from build123d import *

# Parameters (mm, degrees)
BOSS_EXTRUDE1_DEPTH             = 24
SKETCH2_R                       = 4.125
BOSS_EXTRUDE2_DEPTH             = 10
CUT_EXTRUDE1_START              = -24
CUT_EXTRUDE1_DEPTH              = 1.5
CIRPATTERN1_COUNT               = 2
CIRPATTERN1_ANGLE               = 10
CIRPATTERN1_THE_OTHER_WAY_COUNT = 2
CIRPATTERN1_THE_OTHER_WAY_ANGLE = 10


with BuildPart() as part:
    # Sketch1 → Boss-Extrude1 (new body)
    with BuildSketch(Plane(origin=(0, 0, 0), x_dir=(1, 0, 0), z_dir=(0, 1, 0))):
        with BuildLine():
            ThreePointArc((-16.361099339, -0.997559555), (0, -2.429428688), (16.361258496, -0.999379302))
            ThreePointArc((16.361258496, -0.999379302), (19.819023, 3.925881002), (14.885248975, 7.371486655))
            ThreePointArc((14.885248975, 7.371486655), (0, 6.070571326), (-14.885089829, 7.373306345))
            ThreePointArc((-14.885089829, 7.373306345), (-19.808527535, 3.92587815), (-16.361099339, -0.997559555))
        make_face()
    extrude(amount=BOSS_EXTRUDE1_DEPTH)

    # Sketch2 → Boss-Extrude2 (add)
    with BuildSketch(Plane.XZ):
        with Locations(Location((-15.623094584, -3.187873395, 0), (0, 0, 90))):
            Circle(SKETCH2_R)
        with Locations(Location((15.633577289, -3.187873997, 0), (0, 0, 90))):
            Circle(SKETCH2_R)
    extrude(amount=BOSS_EXTRUDE2_DEPTH)

    # Sketch4 → Cut-Extrude1 (cut)
    with BuildSketch(Plane.XZ.offset(CUT_EXTRUDE1_START)):
        with BuildLine():
            Line((-2.1, 2.405913745), (-2.1, -6.140590357))
            ThreePointArc((-2.1, -6.140590357), (-0.000388897, -6.081612393), (2.1, -6.096161069))
            Line((2.1, -6.096161069), (2.1, 2.406147372))
            ThreePointArc((2.1, 2.406147372), (-3.4179e-05, 3.020482466), (-2.1, 2.405913745))
        make_face()
    cut_extrude1 = extrude(amount=CUT_EXTRUDE1_DEPTH, mode=Mode.SUBTRACT)

    # CirPattern1: Cut-Extrude1 ×2 about axis
    cirpattern1_axis = Axis((0.005241406, 24, -91.820571166), (0, 1, 0))
    for i in range(1, CIRPATTERN1_COUNT):
        add(cut_extrude1.rotate(cirpattern1_axis, i * CIRPATTERN1_ANGLE / (CIRPATTERN1_COUNT - 1)), mode=Mode.SUBTRACT)

    # CirPattern1 the other way: Cut-Extrude1 ×2 about axis
    cirpattern1_the_other_way_axis = Axis((0.005241406, 24, -91.820571166), (0, -1, 0))
    for i in range(1, CIRPATTERN1_THE_OTHER_WAY_COUNT):
        add(cut_extrude1.rotate(cirpattern1_the_other_way_axis, i * CIRPATTERN1_THE_OTHER_WAY_ANGLE / (CIRPATTERN1_THE_OTHER_WAY_COUNT - 1)), mode=Mode.SUBTRACT)


solid = part.part
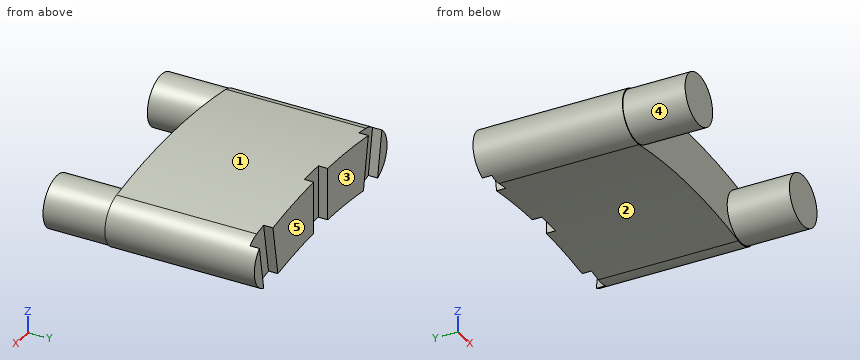
Input: part model. Units: mm. Frame: model coordinates. Face numbers are marked on the shaded views. A direction names the side the tool comes from. Give positions to 0.01 mm unless a question says otherwise; leave off trailing zeros. Write each loop counter-clockwise with the first axis right and the second up, starting at its lowest first coordinate (ties: lowest second). Pieces come first, ordered by that corner, then holes.
Q1. Section C-C, the plane y = -1. Output: boundary loops of the cut face in (x, z) (3 decimals), plus the area to 3 significant figures.
Q2. Section A-A, the plane z = -5. Output: boundary loops of the cut face in (x, y), plus the area to 3 significant figures.
Q3. First-contact query: P1, Ø1, axis at x = 3, y = 6, coming from the -Z side; P2, Ø1, axis at y = 1.5, z = -2, coming from the +X side; P3, Ø12, axis at x = -1.5, y = 8.5, coming from the -Z side. Flat tips, straight axial feed; report the tip coordinate or a pass-through.
Q4. Section B-B, the plane x = 12. Output: boundary loops of the cut face in (y, z).
Q5. Set-up query: the marked faces 4 and 5. Return all of +Z, -Z, +X, -X, +Y, -Y with unobstructed straight access to the full face (end or side cutting, diameter ignored); none if empty.
Q6. Material intervals for probe 1 along Y at (x, z) = (-4, -0.5); probe 2 along Y at (x, z) = (-14, -4.25); probe 3 along X at (y, z) = (-5, -6.75), sorted ascending.
Q7. Pull-direction query (X, two-part tool) for the marked faces 1, 2 and 3; classes: pulls with the +X half, pulls with the -X half, needs draft (parallel to the pull), parting line crosses it, or undercut.
Q8. Section D-D, the plane z = -1. Output: boundary loops of the cut face in (x, y).
Filled in:
1. outline: circle Ø8.25 at (-15.623, -3.188); circle Ø8.25 at (15.634, -3.188)
1. area: 107 mm2
2. outline: (-19.47, 0) - (-19.33, 0) - (-19.33, -10) - (-11.92, -10) - (-11.92, 0) - (11.93, 0) - (11.93, -10) - (19.34, -10) - (19.34, 0) - (19.48, 0) - (19.48, 24) - (17.44, 24) - (17.44, 22.5) - (13.18, 22.5) - (13.18, 24) - (2.1, 24) - (2.1, 22.5) - (-2.1, 22.5) - (-2.1, 24) - (-13.18, 24) - (-13.18, 22.5) - (-17.44, 22.5) - (-17.44, 24) - (-19.47, 24) - close
2. area: 1,060 mm2
3. P1: stops at z = -6.14
3. P2: stops at x = 19.83
3. P3: stops at z = -6.4
4. outline: (-10, -5.14) - (0, -5.14) - (0, -6.91) - (24, -6.91) - (24, 1.66) - (0, 1.66) - (0, -1.24) - (-10, -1.24) - close
5. face 4: -Y
5. face 5: +Z, -Z, +X, -X, +Y
6. probe 1: y = 0 to 24
6. probe 2: y = -10 to 22.5
6. probe 3: x = -17.7 to -13.54, 13.55 to 17.71
7. face 1: parting line crosses it
7. face 2: undercut
7. face 3: needs draft
8. outline: (-19.27, 0) - (-19.12, 0) - (-19.12, -10) - (-12.13, -10) - (-12.13, 0) - (12.14, 0) - (12.14, -10) - (19.13, -10) - (19.13, 0) - (19.28, 0) - (19.28, 24) - (18.15, 24) - (18.15, 22.5) - (13.88, 22.5) - (13.88, 24) - (2.1, 24) - (2.1, 22.5) - (-2.1, 22.5) - (-2.1, 24) - (-13.88, 24) - (-13.88, 22.5) - (-18.15, 22.5) - (-18.15, 24) - (-19.27, 24) - close
